```python
from build123d import *

# Parameters (mm, degrees)
SKETCH1_R           = 25
BOSS_EXTRUDE1_DEPTH = 2.5
SKETCH3_R           = 2.5
BOSS_EXTRUDE3_DEPTH = 7.5
SKETCH5_R           = 3.75
CUT_EXTRUDE1_DEPTH  = 37.742346142


with BuildPart() as part:
    # Sketch1 → Boss-Extrude1 (new, symmetric)
    with BuildSketch(Plane.XY):
        Circle(SKETCH1_R)
    extrude(amount=BOSS_EXTRUDE1_DEPTH, both=True)

    # Sketch3 → Boss-Extrude3 (add)
    with BuildSketch(Plane.XY):
        with Locations(Location((0, 22.5, 0), (0, 0, 90))):
            Circle(SKETCH3_R)
        with BuildLine():
            ThreePointArc((-11.505168712, 9.624504813), (0, -15), (11.505168712, 9.624504813))
            ThreePointArc((11.505168712, 9.624504813), (0, 6.8197992), (-11.505168712, 9.624504813))
        make_face()
    extrude(amount=BOSS_EXTRUDE3_DEPTH)

    # Sketch5 → Cut-Extrude1 (cut, through all)
    with BuildSketch(Plane.XY.offset(7.5)):
        Circle(SKETCH5_R)
    extrude(amount=-CUT_EXTRUDE1_DEPTH, mode=Mode.SUBTRACT)


solid = part.part
```
Work out the finished part from the listing and answer in its coordinate system (mm). A direction names the side the tool comes from. Coordinates: 2 decimals unless noted, no trailing zeros. Order: outer loops, then holes, each group sorted by start corner. A loop starts at its lowest first (then second) coordinate and runs counter-clockwise, first axis right, second up. Notation, with made-up numbers: (69.5, 74) - (100.5, 74) arc R10 cw to (100.5, 91) - close; hole circle Ø4 at (52.25, 22.5). An arc over 180 degrees is marked (long way). Answer as a JSON object with one key per item and string values.
1. Consider line 1 (Y direction, x = 0, z = 0.25); line 2 (Z direction, x = 3, y = 8); line 3 (Y direction, x = -1, z = 3.5). Determine where each line is inside the solid, lowest interval first.
Output values:
{"line 1": "y = -25 to -3.75, 3.75 to 25", "line 2": "z = -2.5 to 2.5", "line 3": "y = -14.97 to -3.61, 3.61 to 6.84, 20.21 to 24.79"}
2. Find section A-A on y = 0. Determine the outline of the cut face in (x, z).
Output values:
{"outline": "(-25, -2.5) - (-3.75, -2.5) - (-3.75, 7.5) - (-15, 7.5) - (-15, 2.5) - (-25, 2.5) - close; (3.75, -2.5) - (25, -2.5) - (25, 2.5) - (15, 2.5) - (15, 7.5) - (3.75, 7.5) - close"}
3. Find section B-B on z = 4. Determine the outline of the cut face in (x, y), plus the area to 3 significant figures.
Output values:
{"outline": "(-11.51, 9.62) arc R15 ccw (long way) to (11.51, 9.62) arc R25 cw to start; circle Ø5 at (0, 22.5); hole circle Ø7.5 at (0, 0)", "area": "553 mm²"}
4. Each of these flat-tipped pins is pushed along its axis until it touches: P1, Ø2, axis at y = 2, z = 4, coming from the +X side; P2, Ø2, axis at y = 5, z = 1.5, coming from the -X side; P3, Ø2, axis at y = 10.5, z = 0, coming from the +X side. Where does it stop, or does it pass through?
Output values:
{"P1": "stops at x = 14.97", "P2": "stops at x = -24.68", "P3": "stops at x = 23.12"}
5. Find section D-D on y = 8.5. Determine the outline of the cut face in (x, z).
Output values:
{"outline": "(-23.51, -2.5) - (23.51, -2.5) - (23.51, 2.5) - (12.36, 2.5) - (12.36, 7.5) - (9.01, 7.5) - (9.01, 2.5) - (-9.01, 2.5) - (-9.01, 7.5) - (-12.36, 7.5) - (-12.36, 2.5) - (-23.51, 2.5) - close"}
6. The mould has two halves that part along Y. Classify faces 3 (the face through (0, -5, 7.5)), 4 (the face through (23.846, 7.509, 0.035)), 5 (the face through (0.17, 6.82, 4.96)): +Y half, -Y half, draft (parallel to the pull), parting line (faces both ways), or undercut.
Output values:
{"face 3": "draft", "face 4": "parting line", "face 5": "undercut"}
7. Find section C-C on x = -9.5. Determine the outline of the cut face in (y, z).
Output values:
{"outline": "(-23.12, -2.5) - (23.12, -2.5) - (23.12, 2.5) - (8.7, 2.5) - (8.7, 7.5) - (-11.61, 7.5) - (-11.61, 2.5) - (-23.12, 2.5) - close"}
8. A tool of negligible diameter and unlimited length cuts with its end or side. For faces 1 (the face through (0, -5, -2.5)), 2 (the face through (0, 11, 2.5)), from which of +Z, -Z, +X, -X, +Y, -Y can it reach the whole face along a straight path? Write none if from no direction.
Output values:
{"face 1": "-Z, +X, -X, +Y, -Y", "face 2": "+Z"}
